Part model, mm, in its own coordinate system. A direction names the side the tool comes from. Give positions to 0.01 mm unless a question says otherwise; leave off trailing zeros. Order: outer loops, then holes, each group sorted by start corner. A loop starts at its lowest first (then second) coordinate and runs counter-clockwise, first axis right, second up.
from build123d import *

# Parameters (mm, degrees)
SKETCH1_R           = 1.1
BOSS_EXTRUDE1_DEPTH = 4.5
SKETCH2_R           = 3
CUT_EXTRUDE2_DEPTH  = 10
CUT_EXTRUDE4_START  = -6
CUT_EXTRUDE4_DEPTH  = 20.401771592
CUT_EXTRUDE6_DEPTH  = 26.401771592
FILLET4_R           = 3
FILLET1_R           = 0.5
SKETCH5_R           = 1.75
CUT_EXTRUDE5_DEPTH  = 1


with BuildPart() as part:
    # Sketch1 → Boss-Extrude1 (new body)
    with BuildSketch(Plane.XY):
        with BuildLine():
            Line((-17, 7), (0, 7))
            ThreePointArc((0, 7), (7, 0), (0, -7))
            Line((0, -7), (-17, -7))
            Line((-17, -7), (-17, 7))
        make_face()
        with Locations((-14, 3.5)):
            Circle(SKETCH1_R, mode=Mode.SUBTRACT)
        with Locations(Location((-14, -3.5, 0), (0, 0, 180))):
            Circle(SKETCH1_R, mode=Mode.SUBTRACT)
    extrude(amount=BOSS_EXTRUDE1_DEPTH)

    # Sketch2 → Cut-Extrude2 (cut)
    with BuildSketch(Plane(origin=(0, 0, 0), x_dir=(-1, 0, 0), z_dir=(0, 0, -1))):
        Circle(SKETCH2_R)
    extrude(amount=-CUT_EXTRUDE2_DEPTH, mode=Mode.SUBTRACT)

    # Sketch7 → Cut-Extrude4 (cut, through all)
    with BuildSketch(Plane.ZY.offset(17).offset(CUT_EXTRUDE4_START)):
        Polygon((2.8, 5.55), (0.6, 5.55), (0.6, 0), (4.5, 0), (4.5, 4.95), (3.4, 4.95), align=None)
        Polygon((4.5, 0), (0.6, 0), (0.6, -5.55), (2.8, -5.55), (3.4, -4.95), (4.5, -4.95), align=None)
    extrude(amount=-CUT_EXTRUDE4_DEPTH, mode=Mode.SUBTRACT)

    # Sketch8 → Cut-Extrude6 (cut, through all)
    with BuildSketch(Plane.ZY.offset(17)):
        with BuildLine():
            Line((3.2, 1.363340016), (3.2, -1.363340016))
            ThreePointArc((3.2, -1.363340016), (3.404046985, -1.855953015), (3.896659984, -2.06))
            Line((3.896659984, -2.06), (4.5, -2.06))
            Line((4.5, -2.06), (4.5, 2.06))
            Line((4.5, 2.06), (3.896659984, 2.06))
            ThreePointArc((3.896659984, 2.06), (3.404046985, 1.855953015), (3.2, 1.363340016))
        make_face()
    extrude(amount=-CUT_EXTRUDE6_DEPTH, mode=Mode.SUBTRACT)

    # Fillet4
    fillet4_edges = [part.edges().sort_by_distance(p)[0] for p in [
        (-17, -7, 2.25),
        (-17, 7, 2.25),
    ]]
    fillet(fillet4_edges, radius=FILLET4_R)

    # Fillet1
    fillet1_edges = [part.edges().sort_by_distance(p)[0] for p in [
        (-7, 7, 0),
        (7, 0, 0),
        (-17, 0, 0),
        (-7, -7, 0),
        (-16.121320344, -6.121320344, 0),
        (-16.121320344, 6.121320344, 0),
    ]]
    fillet(fillet1_edges, radius=FILLET1_R)

    # Sketch5 → Cut-Extrude5 (cut)
    with BuildSketch(Plane.XY):
        with Locations((-14, 3.5)):
            Circle(SKETCH5_R)
        with Locations((-14, -3.5)):
            Circle(SKETCH5_R)
    extrude(amount=CUT_EXTRUDE5_DEPTH, mode=Mode.SUBTRACT)


solid = part.part
Item 1: Band-saw the part on B-B on x = -0.75. List the corners of the cut face in (y, z), plus the area to 3 significant figures.
Item 2: Band-saw the part on A-A on z = 1.4. List the corners of the cut face in (x, y).
Item 3: Pull direction Y, two halves, no side cores. Call faces 4 (the face through (-5, 0, 0)), 5 (the face through (-3, 5.55, 2)), 6 (the face through (-7, 7, 2)): released by +Y, released by -Y, zero draft, split by the parting line, or undercut.
Item 4: Band-saw the part on C-C on x = -11.5. List the corners of the cut face in (y, z).
Item 5: Drill centre lines: probe 1 along Y at (x, z) = (-14, 1.95); probe 2 along Y at (x, z) = (-14, 0.45); probe 3 along Y at (x, z) = (0.25, 2.75). Where is each one in solid material? Low to high.
Item 6: Drop flat-ended pins along their axis: P1, Ø1.4, axis at x = -13.5, y = 0.5, coming from the +Z side; P2, Ø1, axis at y = 4, z = 2.5, coming from the +X side; P3, Ø4.5, axis at x = -14, y = 3.5, coming from the +Z side; P4, Ø0.5, axis at x = -14.5, z = 4, coming from the +Y side. Give the stop position or say it passes through.
Item 7: Band-saw the part on D-D on y = -2.75. Give the number of separate pieces and of enclosed holes in the cut face, plus the area to 3 significant figures.
Item 8: Which spindle directions (+Z, -Z, +X, -X, +Y, -Y) get a long thin tool onto all of the face, cutting with end or side? Do faces 1 (the face through (-3, -4.95, 4)), 2 (the face through (-3, -5.55, 2)), 3 (the face through (-14, 2, 1)). Say none if no direction does.
Working result:
1. outline: (-7, 0.5) arc R0.5 ccw to (-6.5, 0) - (-2.9, 0) - (-2.9, 0.6) - (-5.55, 0.6) - (-5.55, 2.8) - (-4.95, 3.4) - (-4.95, 4.5) - (-7, 4.5) - close; (2.9, 0) - (6.5, 0) arc R0.5 ccw to (7, 0.5) - (7, 4.5) - (4.95, 4.5) - (4.95, 3.4) - (5.55, 2.8) - (5.55, 0.6) - (2.9, 0.6) - close
1. area: 17.8 mm2
2. outline: (-17, -4) arc R3 ccw to (-14, -7) - (0, -7) arc R7 ccw to (4.27, -5.55) - (-11, -5.55) - (-11, 5.55) - (4.27, 5.55) arc R7 ccw to (0, 7) - (-14, 7) arc R3 ccw to (-17, 4) - close; hole circle Ø2.2 at (-14, -3.5); hole circle Ø2.2 at (-14, 3.5)
3. face 4: zero draft
3. face 5: undercut
3. face 6: released by +Y
4. outline: (-7, 0.5) arc R0.5 ccw to (-6.5, 0) - (6.5, 0) arc R0.5 ccw to (7, 0.5) - (7, 4.5) - (2.06, 4.5) - (2.06, 3.9) arc R0.7 cw to (1.36, 3.2) - (-1.36, 3.2) arc R0.7 cw to (-2.06, 3.9) - (-2.06, 4.5) - (-7, 4.5) - close
5. probe 1: y = -7 to -4.6, -2.4 to 2.4, 4.6 to 7
5. probe 2: y = -7 to -5.25, -1.75 to 1.75, 5.25 to 7
5. probe 3: y = -7 to -5.55, 5.55 to 7
6. P1: stops at z = 3.2
6. P2: stops at x = -11
6. P3: stops at z = 4.5
6. P4: stops at y = 6.99
7. separate pieces: 3
7. enclosed holes: 0
7. area: 27.1 mm2
8. face 1: +Z, +X
8. face 2: +X
8. face 3: -Z
